Autodesk Inventor part; units mm, degrees
ref_plane "YZ Plane" through (0, 0, 0) normal (1, 0, 0) x (0, 1, 0)
ref_plane "XZ Plane" through (0, 0, 0) normal (0, 1, 0) x (-1, 0, 0)
ref_plane "XY Plane" through (0, 0, 0) normal (0, 0, 1) x (1, 0, 0)
sketch "Sketch1" plane through (0, 0, 0) normal (0, 1, 0) x (-1, 0, 0)
  line L0 (0, 0) -> (12.7, 0)
  line L1 (12.7, 0) -> (12.7, 63.5)
  line L2 (12.7, 63.5) -> (0, 63.5)
  line L3 (0, 63.5) -> (0, 0)
  circle A0 centre (6.35, 6.35) radius 2.5797
  circle A1 centre (6.35, 57.15) radius 2.5797
  circle A2 centre (6.35, 57.15) radius 6.35
  circle A3 centre (6.35, 6.35) radius 6.35
  dimension "d0" = 12.7
  dimension "d2" = 6.35
  dimension "d3" = 6.35
  dimension "d4" = 5.1594
  dimension "d5" = 6.35
  dimension "d6" = 5.1594
  dimension "d7" = 6.35
  dimension "d43" = 50.8
extrude "Extrusion1" add sketch "Sketch1" along normal blind 25.4
sketch "Sketch4" plane through (0, 0, 63.5) normal (1, 0, 0) x (0, 0, -1)
  circle A0 centre (31.75, 12.7) radius 3.175
  line L0 (0, 0) -> (0, 25.4)
  line L1 (0, 0) -> (63.5, 0)
  circle A1 centre (31.75, 12.7) radius 7.62
  dimension "d30" = 31.75
  dimension "d31" = 12.7
  dimension "d32" = 6.35
  dimension "d37" = 15.24
  dimension "d42" = 63.5
extrude "Extrusion4" cut sketch "Sketch4" against normal blind 12.7 contours A0 | A1
fillet "Fillet1" radius 3.175 4 edges at (-12.7, 25.4, 31.75) (0, 25.4, 31.75) (0, 0, 31.75) (-12.7, 0, 31.75)
fillet "Fillet2" radius 3.175 16 edges at (-0.9299, 24.4701, 63.5) (-6.35, 25.4, 63.5) (-11.7701, 24.4701, 63.5) (-12.7, 12.7, 63.5) (-11.7701, 0.9299, 63.5) (-6.35, 0, 63.5) (-0.9299, 0.9299, 63.5) (0, 12.7, 63.5) (-0.9299, 24.4701, 0) (-6.35, 25.4, 0) (-11.7701, 24.4701, 0) (-12.7, 12.7, 0) (-11.7701, 0.9299, 0) (-6.35, 0, 0) (-0.9299, 0.9299, 0) (0, 12.7, 0)
extrude "Extrusion5" add sketch "Sketch4" against normal blind 9.525
extrude "Extrusion6" cut sketch "Sketch4" against normal blind 3.175
equation "\"d30\" = 0.5 * d42"
properties part number "piston connection"
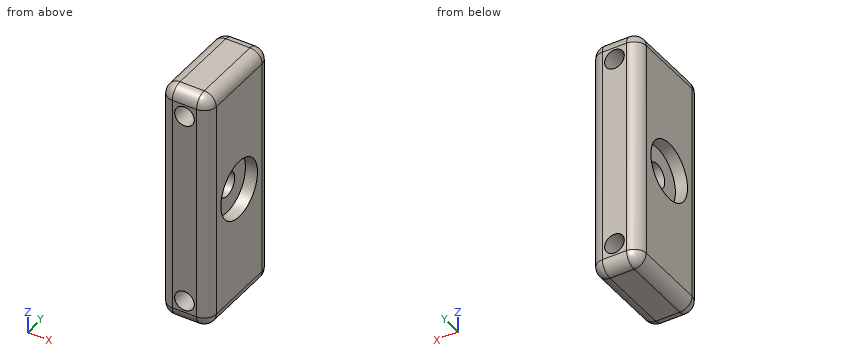
Work out the finished part from the listing and answer in its coordinate system (mm). Give positions to 0.01 mm unless a question says otherwise; leave off trailing zeros. Order: outer loops, then holes, each group sorted by start corner. A loop starts at its lowest first (then second) coordinate and runs counter-clockwise, first axis right, second up. Notation, with made-up numbers: M 1.25,89 L 27.25,89 A6 ccw 27.25,100 Z; hole C -21,69.5 d1. An arc over 180 degrees is marked long. Return JSON: item names as keys, results as strings.
Q1. Each of these flat-tipped pins is pushed along its axis until it touches: pin 1 (9 mm diameter, centred on y = 12.7, z = 31.75, fed in from -X) (3 decimals); pin 2 (4.5 mm diameter, centred on y = 12.5, z = 29, fed in from +X) (3 decimals); pin 3 (3 mm diameter, centred on x = -6.35, z = 57.15, fed in from -Y). Where does it stop, or does it pass through?
Answer below:
{"pin 1": "stops at x = -9.525", "pin 2": "stops at x = -3.175", "pin 3": "passes through"}
Q2. Find the intervals of material crossed by line 1 along Z through (x, y) = (-3.5, 12.5); line 2 along Z through (x, y) = (-7.25, 18); line 3 along Z through (x, y) = (-6.35, 8), in increasing order. Write a range as [from, to].
Answer below:
{"line 1": "z = [0, 28.58], [34.92, 63.5]", "line 2": "z = [0, 3.93], [8.77, 54.73], [59.57, 63.5]", "line 3": "z = [0, 3.77], [8.93, 54.57], [59.73, 63.5]"}
Q3. Find section C-C, the plane x = -5. Write down the section's boundary in (y, z) (3 decimals).
Answer below:
{"outline": "M 0,3.175 A3.175 ccw 3.175,0 L 22.225,0 A3.175 ccw 25.4,3.175 L 25.4,4.152 L 0,4.152 Z; M 0,8.548 L 25.4,8.548 L 25.4,54.952 L 0,54.952 Z; M 0,59.348 L 25.4,59.348 L 25.4,60.325 A3.175 ccw 22.225,63.5 L 3.175,63.5 A3.175 ccw 0,60.325 Z; hole C 12.7,31.75 d6.35"}
Q4. Find section D-D, the plane z = 40. Write down the section's boundary in (x, y) (3 decimals).
Answer below:
{"outline": "M -12.7,3.175 A3.175 ccw -9.525,0 L -3.175,0 A3.175 ccw 0,3.175 L 0,22.225 A3.175 ccw -3.175,25.4 L -9.525,25.4 A3.175 ccw -12.7,22.225 Z"}
Q5. Find section A-A, the plane y = 12.7. Write down the section's boundary in (x, z) (3 decimals), and give its area (3 significant figures).
Answer below:
{"outline": "M -12.7,3.175 A3.175 ccw -9.525,0 L -3.175,0 A3.175 ccw 0,3.175 L 0,24.13 L -3.175,24.13 L -3.175,28.575 L -9.525,28.575 L -9.525,24.13 L -12.7,24.13 Z; M -12.7,39.37 L -9.525,39.37 L -9.525,34.925 L -3.175,34.925 L -3.175,39.37 L 0,39.37 L 0,60.325 A3.175 ccw -3.175,63.5 L -9.525,63.5 A3.175 ccw -12.7,60.325 Z; hole C -6.35,6.35 d5.159; hole C -6.35,57.15 d5.159", "area": "619 mm^2"}
Q6. Find section B-B, the plane z = 57.15. Write down the section's boundary in (x, y) (3 decimals).
Answer below:
{"outline": "M -12.7,3.175 A3.175 ccw -9.525,0 L -8.93,0 L -8.93,25.4 L -9.525,25.4 A3.175 ccw -12.7,22.225 Z; M -3.77,0 L -3.175,0 A3.175 ccw 0,3.175 L 0,22.225 A3.175 ccw -3.175,25.4 L -3.77,25.4 Z"}
